For this review, take the finished solid that the model builds, in its own axes (mm). A direction names the side the tool comes from. Coordinates: 2 decimals unless noted, no trailing zeros. Write each loop counter-clockwise with the first axis right and the second up, starting at its lowest first coordinate (ties: lowest second). Pieces come first, ordered by that corner, then holes.
```python
from build123d import *

# Parameters (mm, degrees)
SKETCH1_W           = 140
SKETCH1_H           = 140
SKETCH1_R           = 1.4
SKETCH1_R_2         = 1.15
SKETCH1_R_3         = 2
SKETCH1_R_4         = 1.65
SKETCH1_W_2         = 14
SKETCH1_H_2         = 62
SKETCH1_W_3         = 3.175
SKETCH1_H_3         = 12
SKETCH1_W_4         = 12
SKETCH1_H_4         = 3.175
BOSS_EXTRUDE1_DEPTH = 3.175
FILLET1_R           = 10


with BuildPart() as part:
    # Sketch1 → Boss-Extrude1 (new body)
    with BuildSketch(Plane(origin=(0, 0, 0), x_dir=(1, 0, 0), z_dir=(0, 1, 0))):
        Rectangle(SKETCH1_W, SKETCH1_H)
        with Locations((29, 4)):
            Circle(SKETCH1_R, mode=Mode.SUBTRACT)
        with Locations((29, -19.05)):
            Circle(SKETCH1_R, mode=Mode.SUBTRACT)
        with Locations((-29, -19.05)):
            Circle(SKETCH1_R, mode=Mode.SUBTRACT)
        with Locations((-29, 4)):
            Circle(SKETCH1_R, mode=Mode.SUBTRACT)
        with Locations((42.225, -20)):
            Circle(SKETCH1_R_2, mode=Mode.SUBTRACT)
        with Locations((42.225, -38)):
            Circle(SKETCH1_R_2, mode=Mode.SUBTRACT)
        with Locations((-42.225, -38)):
            Circle(SKETCH1_R_2, mode=Mode.SUBTRACT)
        with Locations((-42.225, -20)):
            Circle(SKETCH1_R_2, mode=Mode.SUBTRACT)
        with Locations((20, 57.5)):
            Circle(SKETCH1_R_3, mode=Mode.SUBTRACT)
        with Locations((-20, 57.5)):
            Circle(SKETCH1_R_3, mode=Mode.SUBTRACT)
        with Locations((62.928932188, -62.928932188)):
            Circle(SKETCH1_R_4, mode=Mode.SUBTRACT)
        with Locations((62.928932188, 62.928932188)):
            Circle(SKETCH1_R_4, mode=Mode.SUBTRACT)
        with Locations((-62.928932188, -62.928932188)):
            Circle(SKETCH1_R_4, mode=Mode.SUBTRACT)
        with Locations((-62.928932188, 62.928932188)):
            Circle(SKETCH1_R_4, mode=Mode.SUBTRACT)
        with Locations((-53.475, -29)):
            Rectangle(SKETCH1_W_2, SKETCH1_H_2, mode=Mode.SUBTRACT)
        with Locations((53.475, -29)):
            Rectangle(SKETCH1_W_2, SKETCH1_H_2, mode=Mode.SUBTRACT)
        with Locations((-65.2375, -14)):
            Rectangle(SKETCH1_W_3, SKETCH1_H_3, mode=Mode.SUBTRACT)
        with Locations((65.2375, -14)):
            Rectangle(SKETCH1_W_3, SKETCH1_H_3, mode=Mode.SUBTRACT)
        with Locations((14, -65.2375)):
            Rectangle(SKETCH1_W_4, SKETCH1_H_4, mode=Mode.SUBTRACT)
        with Locations((-14, -65.2375)):
            Rectangle(SKETCH1_W_4, SKETCH1_H_4, mode=Mode.SUBTRACT)
        with Locations((65.2375, 14)):
            Rectangle(SKETCH1_W_3, SKETCH1_H_3, mode=Mode.SUBTRACT)
        with Locations((14, 65.2375)):
            Rectangle(SKETCH1_W_4, SKETCH1_H_4, mode=Mode.SUBTRACT)
        with Locations((-14, 65.2375)):
            Rectangle(SKETCH1_W_4, SKETCH1_H_4, mode=Mode.SUBTRACT)
        with Locations((-65.2375, 14)):
            Rectangle(SKETCH1_W_3, SKETCH1_H_3, mode=Mode.SUBTRACT)
    extrude(amount=BOSS_EXTRUDE1_DEPTH)

    # Fillet1
    fillet1_edges = [part.edges().sort_by_distance(p)[0] for p in [
        (70, 1.5875, 70),
        (-70, 1.5875, 70),
        (-70, 1.5875, -70),
        (70, 1.5875, -70),
    ]]
    fillet(fillet1_edges, radius=FILLET1_R)


solid = part.part
```
Q1. Add section A-A (z = -57.5). State the section outline as (x, y) points (3 decimals).
Ans:
outline: (-70, 0) - (-22, 0) - (-22, 3.175) - (-70, 3.175) - close; (-18, 0) - (18, 0) - (18, 3.175) - (-18, 3.175) - close; (22, 0) - (70, 0) - (70, 3.175) - (22, 3.175) - close
Q2. Clearance check with flat-ended pins moving along their axes: pin 1 Ø1 at (x, y) = (-64.5, 1.5) entering from +Z; pin 2 Ø3 at (x, z) = (62.93, -62.93) entering from -Y; pin 3 Ø12 at (x, z) = (9.5, -41.5) entering from -Y; pin 4 Ø1.6 at (x, y) = (66, 2.5) entering from +Z. State where each tip first meets the part, or that it passes through.
Ans:
pin 1: stops at z = 69.17
pin 2: passes through
pin 3: stops at y = 0
pin 4: stops at z = 68.54
Q3. Draft analysis for pull direction Z (two halves, no side actions). For faces 3 (the flat face through (-66.825, 2, -14)), 4 (the cylindrical face through (-67.15, 1.61, 66.99)), 5 (the cylindrical face through (-67.15, 1.61, -66.99)), 6 (the flat face through (-70, 2, 1)), state which applies: +Z half, -Z half, draft (parallel to the pull), parting line (faces both ways), or undercut.
Ans:
face 3: undercut
face 4: +Z half
face 5: -Z half
face 6: draft
Q4. Add section B-B (x = -56.5). State the section outline as (y, z) points (3 decimals).
Ans:
outline: (0, -70) - (3.175, -70) - (3.175, -2) - (0, -2) - close; (0, 60) - (3.175, 60) - (3.175, 70) - (0, 70) - close
Q5. Tool access review of faces 1 (the flat face through (20, 2, -65)), 2 (the flat face through (-1, 0, -1)): name each direction out of +Z, -Z, +X, -X, +Y, -Y from which nothing blocks a thin tool from reaching the whole face with its end or side.
Ans:
face 1: +Y, -Y
face 2: +Z, -Z, +X, -X, -Y
Q6. For probe 1 along X at (y, z) = (1.95, 50) (3 decimals); probe 2 along X at (y, z) = (1.8, 38) (3 decimals); probe 3 along Z at (x, y) = (29, 2.15), list the stretches that pass through material, from the lowest coordinate up.
Ans:
probe 1: x = -70 to -60.475, -46.475 to 46.475, 60.475 to 70
probe 2: x = -70 to -60.475, -46.475 to -43.375, -41.075 to 41.075, 43.375 to 46.475, 60.475 to 70
probe 3: z = -70 to -5.4, -2.6 to 17.65, 20.45 to 70
Q7. Add section D-D (y = 0.7). Give the number of separate pieces and of enclosed holes in the cut face, then the cut area to 3 significant figures.
Ans:
separate pieces: 1
enclosed holes: 24
area: 17,400 mm2
Q8. Add section C-C (z = 4.5). State the section outline as (x, y) points (3 decimals), then the cut area to 3 significant figures.
Ans:
outline: (-70, 0) - (-60.475, 0) - (-60.475, 3.175) - (-70, 3.175) - close; (-46.475, 0) - (46.475, 0) - (46.475, 3.175) - (-46.475, 3.175) - close; (60.475, 0) - (70, 0) - (70, 3.175) - (60.475, 3.175) - close
area: 356 mm2
